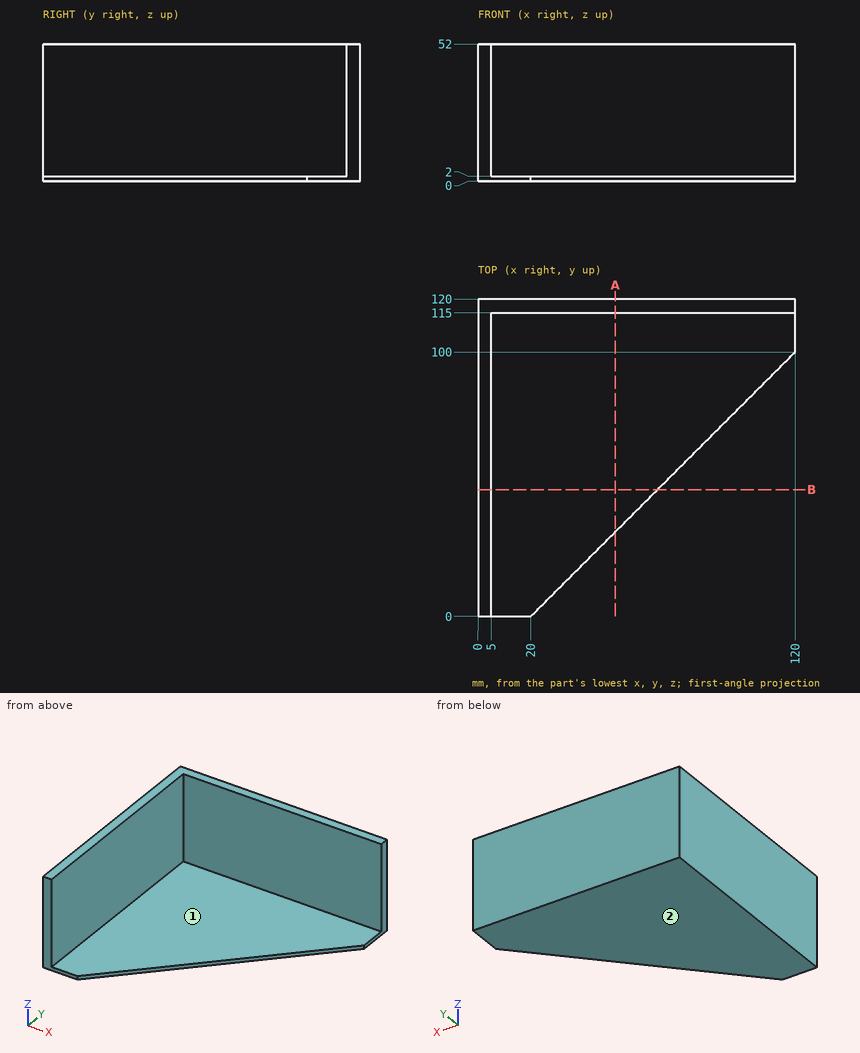
Geometry check sheet. Reference: drawing and pictorial views, mm from the part's lowest x, y, z. A direction names the side the tool comes from. Give positions to 0.01 mm unless a question says otherwise; leave off trailing zeros. Write each loop counter-clockwise with the first axis right and the second up, starting at its lowest first coordinate (ties: lowest second). Pieces come first, ordered by that corner, then holes. Notation, with made-up numbers: (-30, 48) -> (13, 48) arc R22 ccw to (13, 56) -> close; hole circle Ø1 at (78.25, 65). An arc over 180 degrees is marked (long way). One line per item, written item: value. Start each with the question number.
Item 1: Tool access check on the marked faces 1 and 2. Record the directions out of +Z, -Z, +X, -X, +Y, -Y that give a thin tool (end or side, any length) a straight path to the whole face; none if there is none.
Item 2: Material ranges on probe 1 along Y at (x, z) = (37, 16); probe 2 along X at (y, z) = (12.5, 50.5); probe 3 along Z at (x, y) = (38.5, 63), recorded low to high. Write a range as from..to.
Item 3: Section check B-B on y = 48. Record the cut outline in (x, z).
Item 4: Section check A-A on x = 52. Record the cut outline in (y, z).
Item 5: Gauge pin test, flat ends, axial feed: pin 1 (12 mm diameter, centred on y = 102.5, z = 41, fed in from +X); pin 2 (1.5 mm diameter, centred on x = 45, y = 70, fed in from -Z); pin 3 (8 mm diameter, centred on x = 15, y = 91.5, fed in from +Z); pin 4 (1 mm diameter, centred on x = 75, z = 26.5, fed in from -Y). Record the tip position at first contact, or that the pin passes through.
Results list:
1. face 1: +Z, +X, -Y
1. face 2: -Z, +X, -X, +Y, -Y
2. probe 1: 115..120
2. probe 2: 0..5
2. probe 3: 0..2
3. outline: (0, 0) -> (68, 0) -> (68, 2) -> (5, 2) -> (5, 52) -> (0, 52) -> close
4. outline: (32, 0) -> (120, 0) -> (120, 52) -> (115, 52) -> (115, 2) -> (32, 2) -> close
5. pin 1: x = 5
5. pin 2: z = 0
5. pin 3: z = 2
5. pin 4: y = 115
